Verification items for the finished model (mm, model axes). A direction names the side the tool comes from. Round coordinates to 2 decimals unless told otherwise and drop trailing zeros. Order: outer loops, then holes, each group sorted by start corner. A loop starts at its lowest first (then second) coordinate and runs counter-clockwise, first axis right, second up. Notation, with made-up numbers: (78, 53.5) -> (89, 53.5) arc R20 cw to (89, 73.5) -> close; hole circle Ø4 at (29.5, 39.5). An arc over 180 degrees is marked (long way). Answer in a Markdown table with one row per item. Add a question column.
```python
from build123d import *

# Parameters (mm, degrees)
SKETCH1_R           = 2.5
BOSS_EXTRUDE1_DEPTH = 5
SKETCH2_W           = 129.866808808
SKETCH2_H           = 35.545574104
BOSS_EXTRUDE2_DEPTH = 3
SKETCH3_W           = 6.42
SKETCH3_H           = 3
CUT_EXTRUDE1_DEPTH  = 89.860671656
SKETCH4_R           = 4.209133058
SKETCH4_W           = 6.42
SKETCH4_H           = 3
BOSS_EXTRUDE3_DEPTH = 10


with BuildPart() as part:
    # Sketch1 → Boss-Extrude1 (new, symmetric)
    with BuildSketch(Plane.XY):
        with BuildLine():
            Line((50, -1.5), (55, -1.5))
            Line((55, -1.5), (55, 1.5))
            Line((55, 1.5), (-55, 1.5))
            Line((-55, 1.5), (-55, -1.5))
            Line((-55, -1.5), (-50, -1.5))
            Line((-50, -1.5), (-50, -51.5))
            ThreePointArc((-50, -51.5), (-45, -56.5), (-40, -51.5))
            Line((-40, -51.5), (-40, -1.5))
            Line((-40, -1.5), (40, -1.5))
            Line((40, -1.5), (40, -51.5))
            ThreePointArc((40, -51.5), (45, -56.5), (50, -51.5))
            Line((50, -51.5), (50, -1.5))
        make_face()
        with Locations((-45, -51.5)):
            Circle(SKETCH1_R, mode=Mode.SUBTRACT)
        with Locations((45, -51.5)):
            Circle(SKETCH1_R, mode=Mode.SUBTRACT)
    extrude(amount=BOSS_EXTRUDE1_DEPTH, both=True)

    # Sketch2 → Boss-Extrude2 (add)
    with BuildSketch(Plane(origin=(0, 1.5, 0), x_dir=(1, 0, 0), z_dir=(0, 1, 0))):
        Rectangle(SKETCH2_W, SKETCH2_H)
    extrude(amount=-BOSS_EXTRUDE2_DEPTH)

    # Sketch3 → Cut-Extrude1 (cut, through all)
    with BuildSketch(Plane(origin=(0, 1.5, 0), x_dir=(1, 0, 0), z_dir=(0, 1, 0))):
        Rectangle(SKETCH3_W, SKETCH3_H)
    extrude(amount=-CUT_EXTRUDE1_DEPTH, mode=Mode.SUBTRACT)

    # Sketch4 → Boss-Extrude3 (add)
    with BuildSketch(Plane(origin=(0, 1.5, 0), x_dir=(1, 0, 0), z_dir=(0, 1, 0))):
        Circle(SKETCH4_R)
        Rectangle(SKETCH4_W, SKETCH4_H, mode=Mode.SUBTRACT)
    extrude(amount=BOSS_EXTRUDE3_DEPTH)


solid = part.part
```
1) Draft check along X on faces 1 (the face through (44.9, -56.5, 0.1)), 2 (the face through (-45, -29, -5)), 3 (the face through (47.31, -52.46, -0.07)), 4 (the face through (-64.933, 0, 0)). Enter one of: +X half, -X half, draft (parallel to the pull), parting line (faces both ways), or undercut.
2) Cross-section at B-B, the plane x = 45. Record the boundary of the cut face in (y, z).
3) Cross-section at D-D, the plane x = 0. Record the boundary of the cut face in (y, z), and give its area (3 significant figures).
4) Thickness scan on L1, parallel to X at y = -52.5, z = 1.5; L2, parallel to Y at x = 45, z = -1.75; L3, parallel to Y at x = -17, z = 0.5. Record the ranges inside material, lowest first. Write a range as [from, to].
5) Tool access check on faces 5 (the face through (3.21, 5, 0)), 6 (the face through (-50, -26, 0)), 7 (the face through (40, -26, 0)), 8 (the face through (45, -29, -5)), 9 (the face through (45, -29, 5)). Record the directions out of +Z, -Z, +X, -X, +Y, -Y that give a thin tool (end or side, any length) a straight path to the whole face; none if there is none.
6) Cross-section at C-C, the plane y = -46.5. Record the boundary of the cut face in (x, z), and give its area (3 significant figures).
7) Cross-section at A-A, the plane z = 0. Record the boundary of the cut face in (x, y).
8) Depth check by flat-ended pin: P1, Ø1.5, axis at x = -49.5, y = -29.5, coming from the -Z side; P2, Ø11, axis at y = -16.5, z = 1.5, coming from the -X side; P3, Ø0.9, axis at y = 4, z = 0, coming from the -X side. Enter the tip coordinate at first touch or a pass-through.
Results below:
| question | item | result |
|---|---|---|
| 1 | face 1 | undercut |
| 1 | face 2 | draft |
| 1 | face 3 | undercut |
| 1 | face 4 | -X half |
| 2 | outline | (-56.5, -5) -> (-54, -5) -> (-54, 5) -> (-56.5, 5) -> close; (-49, -5) -> (-1.5, -5) -> (-1.5, -17.77) -> (1.5, -17.77) -> (1.5, 17.77) -> (-1.5, 17.77) -> (-1.5, 5) -> (-49, 5) -> close |
| 3 | outline | (-1.5, -17.77) -> (1.5, -17.77) -> (1.5, -4.21) -> (11.5, -4.21) -> (11.5, -1.5) -> (-1.5, -1.5) -> close; (-1.5, 1.5) -> (11.5, 1.5) -> (11.5, 4.21) -> (1.5, 4.21) -> (1.5, 17.77) -> (-1.5, 17.77) -> close |
| 3 | area | 152 mm² |
| 4 | L1 | [-49.9, -47.29], [-42.71, -40.1], [40.1, 42.71], [47.29, 49.9] |
| 4 | L2 | [-56.5, -54], [-49, 1.5] |
| 4 | L3 | [-1.5, 1.5] |
| 5 | face 5 | +Y, -Y |
| 5 | face 6 | +Z, -Z, -X, -Y |
| 5 | face 7 | +Z, -Z, -Y |
| 5 | face 8 | -Z, +X, -X, -Y |
| 5 | face 9 | +Z, +X, -X, -Y |
| 6 | outline | (-50, -5) -> (-40, -5) -> (-40, 5) -> (-50, 5) -> close; (40, -5) -> (50, -5) -> (50, 5) -> (40, 5) -> close |
| 6 | area | 200 mm² |
| 7 | outline | (-64.93, -1.5) -> (-50, -1.5) -> (-50, -51.5) arc R5 ccw to (-40, -51.5) -> (-40, -1.5) -> (-3.21, -1.5) -> (-3.21, 11.5) -> (-4.21, 11.5) -> (-4.21, 1.5) -> (-64.93, 1.5) -> close; (3.21, -1.5) -> (40, -1.5) -> (40, -51.5) arc R5 ccw to (50, -51.5) -> (50, -1.5) -> (64.93, -1.5) -> (64.93, 1.5) -> (4.21, 1.5) -> (4.21, 11.5) -> (3.21, 11.5) -> close; hole circle Ø5 at (-45, -51.5); hole circle Ø5 at (45, -51.5) |
| 8 | P1 | z = -5 |
| 8 | P2 | x = -50 |
| 8 | P3 | x = -4.21 |
